from build123d import *

# Parameters (mm, degrees)
F0_R      = 9
F1_DEPTH  = 0.5
F2_R      = 5
F3_DEPTH  = 8
F4_R      = 2.46
F5_DEPTH  = 6
F6_R      = 5
F7_DEPTH  = 0.5
F8_R      = 5.5
F9_DEPTH  = 1.5
F10_R     = 4
F11_DEPTH = 0.25


with BuildPart() as f1:
    # F0 (on Top) → F1 (new body)
    with BuildSketch(Plane.XY):
        Circle(F0_R)
    extrude(amount=F1_DEPTH)

    # F2 (on face) → F3 (join)
    with BuildSketch(Plane.XY.offset(0.5)):
        Circle(F2_R)
    extrude(amount=F3_DEPTH)

    # F4 (on face) → F5 (cut)
    with BuildSketch(Plane(origin=(0, 0, 0), x_dir=(1, 0, 0), z_dir=(0, 0, -1))):
        Circle(F4_R)
    extrude(amount=-F5_DEPTH, mode=Mode.SUBTRACT)

    # F6 (on face) → F7 (cut)
    with BuildSketch(Plane.XY.offset(8.5)):
        Circle(F6_R)
    extrude(amount=-F7_DEPTH, mode=Mode.SUBTRACT)

    # F8 (on face) → F9 (join)
    with BuildSketch(Plane.XY.offset(0.5)):
        Circle(F8_R)
    extrude(amount=F9_DEPTH)

    # F10 (on face) → F11 (cut)
    with BuildSketch(Plane.XY.offset(8)):
        Circle(F10_R)
    extrude(amount=-F11_DEPTH, mode=Mode.SUBTRACT)


solid = f1.part
Work out the finished part from the listing and answer in its coordinate system (mm). A direction names the side the tool comes from. Coordinates: 2 decimals unless noted, no trailing zeros. Write each loop counter-clockwise with the first axis right and the second up, starting at its lowest first coordinate (ties: lowest second). Pieces come first, ordered by that corner, then holes.
1. For faces 1 (the flat face through (0, 0, 0.5)), 2 (the flat face through (0, 0, 2)), 3 (the flat face through (0, 0, 7.75)), determine the directions among +Z, -Z, +X, -X, +Y, -Y from which every point of the face is accessible in a straight line to the end or side of a thin tool.
Results list:
face 1: -Z
face 2: none
face 3: +Z
2. The part is cut by section D-D, the plane x = 4.5. Write down the section's boundary in (y, z).
Results list:
outline: (-7.79, 0) - (7.79, 0) - (7.79, 0.5) - (3.16, 0.5) - (3.16, 2) - (2.18, 2) - (2.18, 8) - (-2.18, 8) - (-2.18, 2) - (-3.16, 2) - (-3.16, 0.5) - (-7.79, 0.5) - close
3. The part is cut by section C-C, the plane z = 3.5. Write down the section's boundary in (x, y), and give its area (3 significant figures).
Results list:
outline: circle Ø10 at (0, 0); hole circle Ø4.92 at (0, 0)
area: 59.5 mm2
4. For a pull along X with two mould halves and no side action, classify faces 4 (the flat face through (-4, -4, 0.5)), 5 (the cylindrical face through (-1.19, -5.37, 1.24)), 6 (the cylindrical face through (2.272, 0.942, 0.246)) as +X half, -X half, draft (parallel to the pull), parting line (faces both ways), or undercut.
Results list:
face 4: draft
face 5: parting line
face 6: undercut
5. Flat-ended cylindrical pins translate along their axes: pin 1 (1 mm diameter, centred on y = 1, z = 2, fed in from -X); pin 2 (3 mm diameter, centred on x = 3.5, z = 1.5, fed in from +Y); pin 3 (2.5 mm diameter, centred on x = -0.5, y = 0, fed in from +Z). Find the tip coordinate at first contact, or state that the pin passes through.
Results list:
pin 1: stops at x = -5.48
pin 2: stops at y = 8.68
pin 3: stops at z = 7.75
6. Consider line 1 along Z through (x, y) = (-1.5, -1.75); line 2 along Y through (x, z) = (0, 7.8); line 3 along Y through (x, z) = (0, 3.7). Determine where each line is inside the solid, lowest interval first.
Results list:
line 1: z = 0.5 to 2, 6 to 7.75
line 2: y = -5 to -4, 4 to 5
line 3: y = -5 to -2.46, 2.46 to 5
7. The part is cut by section A-A, the plane y = 0. Write down the section's boundary in (x, z).
Results list:
outline: (-9, 0) - (-2.46, 0) - (-2.46, 0.5) - (2.46, 0.5) - (2.46, 0) - (9, 0) - (9, 0.5) - (5.5, 0.5) - (5.5, 2) - (5, 2) - (5, 8) - (4, 8) - (4, 7.75) - (-4, 7.75) - (-4, 8) - (-5, 8) - (-5, 2) - (-5.5, 2) - (-5.5, 0.5) - (-9, 0.5) - close; hole (-2.46, 2) - (2.46, 2) - (2.46, 6) - (-2.46, 6) - close
